Read the model definition and answer for the solid it produces. Units are mm, in the model's axes. Give positions to 0.01 mm unless a question says otherwise; leave off trailing zeros. Order: outer loops, then holes, each group sorted by start corner. A loop starts at its lowest first (then second) coordinate and runs counter-clockwise, first axis right, second up. Notation, with made-up numbers: (-28, 4) - (-12, 4) arc R21 ccw to (-12, 36) - close; hole circle Ø7 at (1, -23). An arc over 180 degrees is marked (long way). Use a Markdown table: item, result. Add a question column.
1. Flat-ended cylindrical pins translate along their axes: P1, Ø10, axis at x = -223, z = -118.5, coming from the -Y side; P2, Ø2.5, axis at x = -208.7, z = -96.67, coming from the -Y side. Find the tip coordinate at first contact, or state that the pin passes through.
2. A cutting plane is placed at A-A on z = -101. Determine the outline of the cut face in (x, y).
3. For a pull along Z with two mould halves and no side action, classify faces 1 (the flat face through (-215, 0, -112)), 2 (the cylindrical face through (-201.5, 1.01, -125.45)), 3 (the cylindrical face through (-200.114, 1.014, -100.942)), 4 (the cylindrical face through (-211.286, 0.986, -118.708)) as released by +Z, released by -Z, zero draft, split by the parting line, or undercut.
4. A cutting plane is placed at C-C on y = 1.1. Determine the outline of the cut face in (x, z), and give its area (3 significant figures).
5. A cutting plane is placed at D-D on x = -215.5. Determine the outline of the cut face in (y, z).
6. A cutting plane is placed at B-B on x = -220. Determine the outline of the cut face in (y, z), and give its area (3 significant figures).
7. Consider L1, parallel to Z at x = -217.75, y = 1.35; L2, parallel to Z at x = -216.5, y = 1.55; L3, parallel to Z at x = -213.75, y = 1.5. Determine where each line is inside the solid, lowest interval first.
```python
from build123d import *

# Parameters (mm, degrees)
SKETCH_1_R      = 1.45
EXTRUDE_1_DEPTH = 2
FILLET_1_R      = 5


with BuildPart() as part:
    # 草图1 → 凸台-拉伸1 (new body)
    with BuildSketch(Plane(origin=(0, 0, 0), x_dir=(1, 0, 0), z_dir=(0, 1, 0))):
        Polygon((-230, 126.877091055), (-230, 98.266220035), (-206.304299333, 87.290817382), (-200, 100.901688402), (-200, 126.877091055), align=None)
        with Locations(Location((-217.77393632, 100.868789323, 0), (0, 0, 270))):
            Circle(SKETCH_1_R, mode=Mode.SUBTRACT)
        with Locations(Location((-208.700022307, 96.665923102, 0), (0, 0, 270))):
            Circle(SKETCH_1_R, mode=Mode.SUBTRACT)
        with Locations(Location((-220, 119.377091055, 0), (0, 0, 270))):
            Circle(SKETCH_1_R, mode=Mode.SUBTRACT)
        with Locations(Location((-210, 119.377091055, 0), (0, 0, 270))):
            Circle(SKETCH_1_R, mode=Mode.SUBTRACT)
    extrude(amount=EXTRUDE_1_DEPTH)

    # 圆角1
    fillet_1_edges = [part.edges().sort_by_distance(p)[0] for p in [
        (-200, 1, -126.877091055),
        (-200, 1, -100.901688402),
        (-206.304299333, 1, -87.290817382),
        (-230, 1, -98.266220035),
        (-230, 1, -126.877091055),
    ]]
    fillet(fillet_1_edges, radius=FILLET_1_R)


solid = part.part
```
Output values:
| question | item | result |
|---|---|---|
| 1 | P1 | y = 0 |
| 1 | P2 | through |
| 2 | outline | (-229.98, 0) - (-219.22, 0) - (-219.22, 2) - (-229.98, 2) - close; (-216.33, 0) - (-200.1, 0) - (-200.1, 2) - (-216.33, 2) - close |
| 3 | face 1 | zero draft |
| 3 | face 2 | released by -Z |
| 3 | face 3 | released by +Z |
| 3 | face 4 | undercut |
| 4 | outline | (-230, -121.88) arc R5 ccw to (-225, -126.88) - (-205, -126.88) arc R5 ccw to (-200, -121.88) - (-200, -102) arc R5 ccw to (-200.46, -99.9) - (-204.2, -91.83) arc R5 ccw to (-210.84, -89.39) - (-227.1, -96.92) arc R5 ccw to (-230, -101.46) - close; hole circle Ø2.9 at (-220, -119.38); hole circle Ø2.9 at (-217.77, -100.87); hole circle Ø2.9 at (-210, -119.38); hole circle Ø2.9 at (-208.7, -96.67) |
| 4 | area | 970 mm² |
| 5 | outline | (0, -126.88) - (2, -126.88) - (2, -91.55) - (0, -91.55) - close |
| 6 | outline | (0, -126.88) - (2, -126.88) - (2, -120.83) - (0, -120.83) - close; (0, -117.93) - (2, -117.93) - (2, -93.63) - (0, -93.63) - close |
| 6 | area | 60.7 mm² |
| 7 | L1 | -126.88 to -102.32, -99.42 to -92.59 |
| 7 | L2 | -126.88 to -101.56, -100.18 to -92.01 |
| 7 | L3 | -126.88 to -90.74 |
